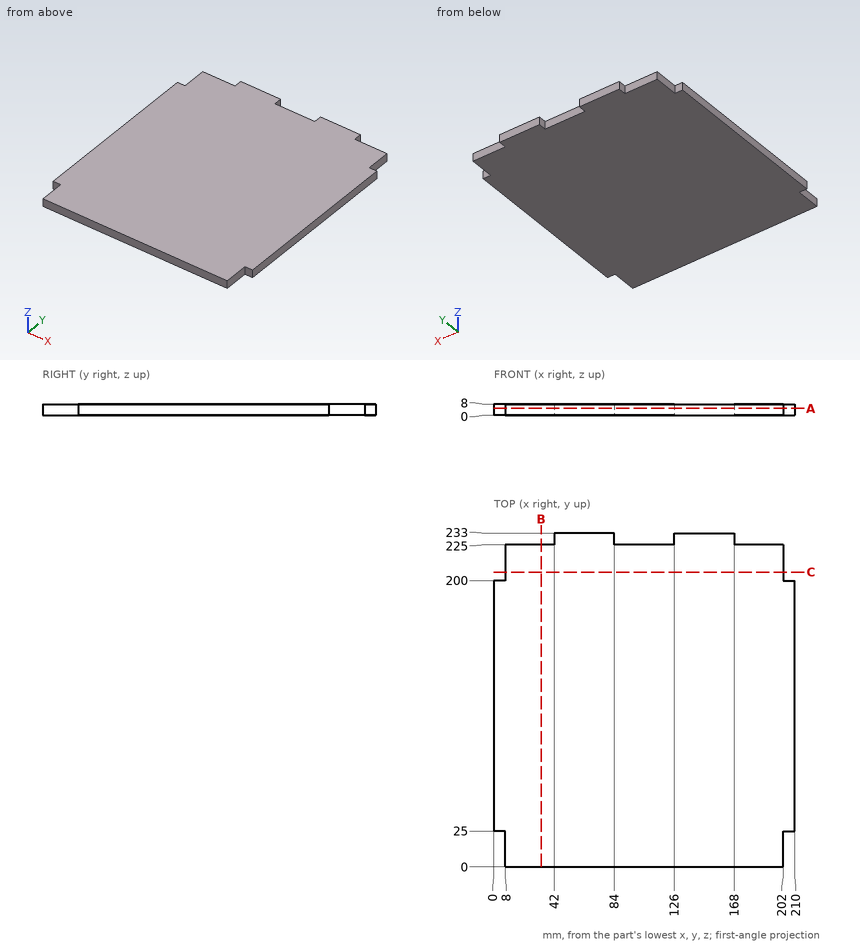
Job drawing, mm, ordinate dimensions from the low corner. One solid piece. Round coordinates to 2 decimals unless told otherwise and drop trailing zeros. Loops run counter-clockwise (first coordinate to the right, second up) from the corner with the lowest first, then second, coordinate; pieces in that order, holes last.
(1) Wall check: line 1 along X through (y, z) = (200.5, 7); line 2 along Y through (x, z) = (32, 2.75). Give the ranges that are in metal, low to high.
(2) Drop flat-ended pins along their axis: pin 1 (8 mm diameter, centred on x = 43.5, y = 67, fed in from -Z); pin 2 (2.5 mm diameter, centred on y = 230.5, z = 5.5, fed in from -X); pin 3 (4 mm diameter, centred on x = 205.5, z = 4.5, fed in from +Y); pin 4 (2.5 mm diameter, centred on y = 218, z = 3, fed in from -X). Give the stop position or say it passes through.
(3) Cut at C-C (y = 206). Give the cut face in (x, z).
(4) Cut at A-A (z = 5). Give the cut face in (x, y).
(5) Cut at B-B (x = 33). Give the cut face in (y, z).
Findings below:
1. line 1: x = 8 to 202
1. line 2: y = 0 to 225
2. pin 1: stops at z = 0
2. pin 2: stops at x = 42
2. pin 3: stops at y = 200
2. pin 4: stops at x = 8
3. outline: (8, 0) - (202, 0) - (202, 8) - (8, 8) - close
4. outline: (0, 25) - (8, 25) - (8, 0) - (202, 0) - (202, 25) - (210, 25) - (210, 200) - (202, 200) - (202, 225) - (168, 225) - (168, 233) - (126, 233) - (126, 225) - (84, 225) - (84, 233) - (42, 233) - (42, 225) - (8, 225) - (8, 200) - (0, 200) - close
5. outline: (0, 0) - (225, 0) - (225, 8) - (0, 8) - close
